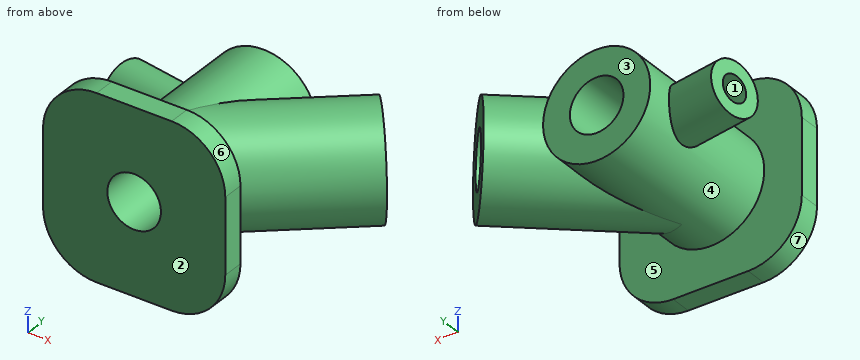
```python
from build123d import *

# Parameters (mm, degrees)
BOSS_EXTRUDE1_DEPTH            = 20
SKETCH3_R                      = 50
BOSS_EXTRUDE2_DEPTH            = 150
SKETCH4_R                      = 25
CUT_EXTRUDE1_DEPTH             = 170
BOSS_EXTRUDE4_REACH            = 259.695
SKETCH6_R                      = 50
CUT_EXTRUDE2_REACH             = 259.695
SKETCH7_R                      = 25
CUT_EXTRUDE2_DIRECTION_2_DEPTH = 50.240387651
BOSS_EXTRUDE5_REACH            = 270.866
SKETCH9_R                      = 25
CUT_EXTRUDE3_REACH             = 270.866
SKETCH10_R                     = 12.5


with BuildPart() as part:
    # Sketch2 → Boss-Extrude1 (new body)
    with BuildSketch(Plane(origin=(0, 0, 0), x_dir=(1, 0, 0), z_dir=(0, 1, 0))):
        with BuildLine():
            Line((35, -85), (-35, -85))
            ThreePointArc((-35, -85), (-70.355339059, -70.355339059), (-85, -35))
            Line((-85, -35), (-85, 35))
            ThreePointArc((-85, 35), (-70.355339059, 70.355339059), (-35, 85))
            Line((-35, 85), (35, 85))
            ThreePointArc((35, 85), (70.355339059, 70.355339059), (85, 35))
            Line((85, 35), (85, -35))
            ThreePointArc((85, -35), (70.355339059, -70.355339059), (35, -85))
        make_face()
    extrude(amount=BOSS_EXTRUDE1_DEPTH)

    # Sketch3 → Boss-Extrude2 (add)
    with BuildSketch(Plane(origin=(0, 20, 0), x_dir=(1, 0, 0), z_dir=(0, 1, 0))):
        Circle(SKETCH3_R)
    extrude(amount=BOSS_EXTRUDE2_DEPTH)

    # Sketch4 → Cut-Extrude1 (cut)
    with BuildSketch(Plane(origin=(0, 170, 0), x_dir=(1, 0, 0), z_dir=(0, 1, 0))):
        Circle(SKETCH4_R)
    extrude(amount=-CUT_EXTRUDE1_DEPTH, mode=Mode.SUBTRACT)

    # Sketch6 → Boss-Extrude4 (add, up to next)
    with BuildSketch(Plane(origin=(147.525591973, 123.788669814, 0), x_dir=(0, 0, -1), z_dir=(0.766044443, 0.64278761, 0)), mode=Mode.PRIVATE) as boss_extrude4_sk1:
        with Locations((0, 44.465063828)):
            Circle(SKETCH6_R)
    boss_extrude4_tool1 = extrude(boss_extrude4_sk1.sketch, amount=-BOSS_EXTRUDE4_REACH, mode=Mode.PRIVATE) - part.part
    add(boss_extrude4_tool1.solids().sort_by_distance((118.944, 157.850885, 0))[0])

    # Sketch7 → Cut-Extrude2 (cut, up to next)
    with BuildSketch(Plane(origin=(147.525591973, 123.788669814, 0), x_dir=(0, 0, -1), z_dir=(0.766044443, 0.64278761, 0)), mode=Mode.PRIVATE) as cut_extrude2_sk1:
        with Locations((0, 44.465063828)):
            Circle(SKETCH7_R)
    cut_extrude2_tool1 = extrude(cut_extrude2_sk1.sketch, amount=-CUT_EXTRUDE2_REACH, mode=Mode.PRIVATE) & part.part
    add(cut_extrude2_tool1.solids().sort_by_distance((118.944, 157.850885, 0))[0], mode=Mode.SUBTRACT)

    # Sketch7 → Cut-Extrude2 direction 2 (cut)
    with BuildSketch(Plane(origin=(147.525591973, 123.788669814, 0), x_dir=(0, 0, -1), z_dir=(0.766044443, 0.64278761, 0))):
        with Locations((0, 44.465063828)):
            Circle(SKETCH7_R)
    extrude(amount=CUT_EXTRUDE2_DIRECTION_2_DEPTH, mode=Mode.SUBTRACT)

    # Sketch9 → Boss-Extrude5 (add, up to next)
    with BuildSketch(Plane(origin=(-118.25391177, 20.851355219, 0), x_dir=(0, 0, -1), z_dir=(0.984807753, -0.173648178, 0)), mode=Mode.PRIVATE) as boss_extrude5_sk1:
        with Locations((0, 109.494521478)):
            Circle(SKETCH9_R)
    boss_extrude5_tool1 = extrude(boss_extrude5_sk1.sketch, amount=BOSS_EXTRUDE5_REACH, mode=Mode.PRIVATE) - part.part
    add(boss_extrude5_tool1.solids().sort_by_distance((-99.240388, 128.682409, 0))[0])

    # Sketch10 → Cut-Extrude3 (cut, up to next)
    with BuildSketch(Plane(origin=(-118.25391177, 20.851355219, 0), x_dir=(0, 0, 1), z_dir=(-0.984807753, 0.173648178, 0)), mode=Mode.PRIVATE) as cut_extrude3_sk1:
        with Locations((0, 109.494521478)):
            Circle(SKETCH10_R)
    cut_extrude3_tool1 = extrude(cut_extrude3_sk1.sketch, amount=-CUT_EXTRUDE3_REACH, mode=Mode.PRIVATE) & part.part
    add(cut_extrude3_tool1.solids().sort_by_distance((-99.240388, 128.682409, 0))[0], mode=Mode.SUBTRACT)


solid = part.part
```
The listing builds one solid part. Answer for the finished solid, in the listing's coordinates (mm). Face numbers are marked on the shaded views. A direction names the side the tool comes from. Coordinates: 2 decimals unless noted, no trailing zeros. Write each loop counter-clockwise with the first axis right and the second up, starting at its lowest first coordinate (ties: lowest second). Pieces come first, ordered by that corner, then holes. Notation, with made-up numbers: (61.25, -7.5) -> (69.25, -7.5) arc R27 cw to (69.25, 16.5) -> close; hole circle Ø9 at (73, -26). An arc over 180 degrees is marked (long way). Write each question's results on one line, items separated by ' | '. Start each with the question number.
1) Flat-ended cylindrical pins translate along their axes: pin 1 Ø16 at (y, z) = (13, -1.5) entering from +X; pin 2 Ø4 at (x, z) = (28.5, -9.5) entering from +Y; pin 3 Ø2 at (x, y) = (64.5, 100.5) entering from +Z; pin 4 Ø10 at (x, z) = (-72.5, 36.5) entering from -Y. Find the tip coordinate at first contact, or state that the pin passes through.
2) Straight lines are drawn through the part: probe 1 along Z at (x, y) = (0, 132); probe 2 along Y at (x, z) = (63, -8); probe 3 along Y at (x, z) = (-46, -36). For each, find the intervals that lie inside material, in ascending order.
3) A cutting plane is placed at A-A (z = 0). Determine the outline of the cut face in (x, y), then the cut area to 3 significant figures.
4) For a pull along Y with two mould halves and no side action, classify the marked faces 1, 2, 3 and 4 as +Y half, -Y half, draft (parallel to the pull), parting line (faces both ways), or undercut.
5) A cutting plane is placed at B-B (x = 58.5). Count the separate pieces of the cut face and the enclosed holes in it, then the cut area to 3 significant figures.
6) A tool of negligible diameter and unlimited length cuts with its end or side. For the marked faces 5, 6 and 7, from which of +Z, -Z, +X, -X, +Y, -Y can it reach the whole face along a straight path? Write none if from no direction.
7) A cutting plane is placed at C-C (z = -59.5). Determine the outline of the cut face in (x, y), then the cut area to 3 significant figures.
Values follow:
1) pin 1: x = 85 | pin 2: y = 170 | pin 3: z = 49.37 | pin 4: y = 0
2) probe 1: -50 to -25, 25 to 50 | probe 2: 0 to 20, 46.48 to 79.99, 141.83 to 175.34 | probe 3: 0 to 20
3) outline: (-103.58, 104.06) -> (-50, 94.61) -> (-50, 20) -> (-85, 20) -> (-85, 0) -> (-25, 0) -> (-25, 102.9) -> (-101.41, 116.37) -> close; (-97.07, 140.99) -> (-25, 128.28) -> (-25, 170) -> (-50, 170) -> (-50, 145.39) -> (-94.9, 153.3) -> close; (25, 0) -> (85, 0) -> (85, 20) -> (50, 20) -> (50, 34.73) -> (151.08, 119.55) -> (135.01, 138.7) -> (25, 46.39) -> close; (25, 111.66) -> (102.87, 177) -> (86.8, 196.15) -> (50, 165.27) -> (50, 170) -> (25, 170) -> close | area: 13,400 mm²
4) face 1: undercut | face 2: -Y half | face 3: +Y half | face 4: undercut
5) separate pieces: 2 | enclosed holes: 1 | area: 10,900 mm²
6) face 5: none | face 6: +Z, +X, -Y | face 7: -Z, -X, +Y, -Y
7) outline: (-78.59, 0) -> (78.59, 0) -> (78.59, 20) -> (-78.59, 20) -> close | area: 3,140 mm²
